```python
from build123d import *

# Parameters (mm, degrees)
F2_DEPTH       = 70
F4_D           = 3.5
F4_CSINK_D     = 7
F4_CSINK_ANGLE = 90


with BuildPart() as f2:
    # F1 (on Front) → F2 (new body)
    with BuildSketch(Plane.XZ):
        with BuildLine():
            Line((0, 3.2153789857), (0, 0))
            Line((0, 0), (41.3793856046, 0))
            Line((41.3793856046, 0), (41.3793856046, 12.0218454194))
            Line((41.3793856046, 12.0218454194), (37.0459675166, 12.0218454194))
            ThreePointArc((37.0459675166, 12.0218454194), (27.4254767926, 4.7506103835), (17.8049860686, 12.0218454194))
            Line((17.8049860686, 12.0218454194), (13.4715679806, 12.0218454194))
            Line((13.4715679806, 12.0218454194), (13.4715679806, 3.2153789857))
            Line((13.4715679806, 3.2153789857), (0, 3.2153789857))
        make_face()
    extrude(amount=F2_DEPTH)

    # F4 (through all)
    with Locations(Plane.XY.offset(3.2153789857)):
        with Locations((6.7357839903, -20), (6.7357839903, -50)):
            CounterSinkHole(F4_D / 2, F4_CSINK_D / 2, counter_sink_angle=F4_CSINK_ANGLE)


solid = f2.part
```
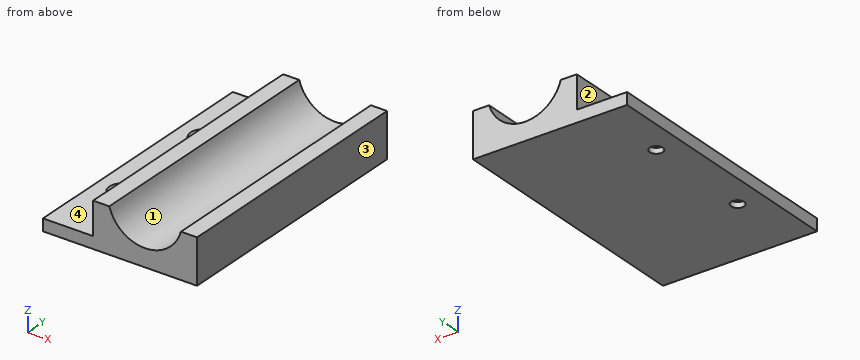
Can you work these out from the model? Positions are in its coordinate system, mm. Face numbers are marked on the shaded views. Round coordinates to 2 decimals unless told otherwise and drop trailing zeros. Loops run counter-clockwise (first coordinate to the right, second up) from the corner with the lowest first, then second, coordinate; pieces in that order, holes last. Notation, with made-up numbers: M -29,78.5 L 28,78.5 A27 cw 28,97.5 Z; hole C 50.5,77.25 d3. An arc over 180 degrees is marked long. Answer in a Markdown table with one row per item.
1. If we section it at C-C, the plane z = 10: Please give me the cut outline in (x, y) (3 decimals).
Established:
| item | result |
|---|---|
| outline | M 13.472,-70 L 18.626,-70 L 18.626,0 L 13.472,0 Z; M 36.225,-70 L 41.379,-70 L 41.379,0 L 36.225,0 Z |
2. If we section it at D-D, the plane x = 24: Please give me the cut outline in (y, z), plus the area to 3 significant figures.
Established:
| item | result |
|---|---|
| outline | M -70,0 L 0,0 L 0,5.36 L -70,5.36 Z |
| area | 375 mm² |
3. If we section it at A-A, the plane y = -20: Please give me the cut outline in (x, z), plus the area to 3 significant figures.
Established:
| item | result |
|---|---|
| outline | M 0,0 L 4.99,0 L 4.99,1.47 L 3.24,3.22 L 0,3.22 Z; M 8.49,0 L 41.38,0 L 41.38,12.02 L 37.05,12.02 A10 cw 17.8,12.02 L 13.47,12.02 L 13.47,3.22 L 10.24,3.22 L 8.49,1.47 Z |
| area | 261 mm² |
4. I'm going to push flat-ended pins straight in: pin 1 Ø4 at (x, y) = (29.5, -51) entering from +Z; pin 2 Ø4.5 at (x, y) = (6.74, -20) entering from +Z; pin 3 Ø4.5 at (y, z) = (-20, 9.5) entering from -X. Where does each tip first touch, or does it pass through?
Established:
| item | result |
|---|---|
| pin 1 | z = 5.62 |
| pin 2 | z = 1.97 |
| pin 3 | x = 13.47 |
5. Please list where these lines run through material, in increasing order: line 1 (X direction, y = -20, z = 0.9); line 2 (Z direction, x = 11, y = -19.5); line 3 (X direction, y = -4.5, z = 3.5). Write a range as from..to.
Established:
| item | result |
|---|---|
| line 1 | 0..4.99, 8.49..41.38 |
| line 2 | 0..3.22 |
| line 3 | 13.47..41.38 |
6. Thinking about a two-plate mould opening in X: for the marked faces 1, 2, 3 and 4, which applies, pulls with the +X half, pulls with the -X half, needs draft (parallel to the pull), parting line crosses it, or undercut?
Established:
| item | result |
|---|---|
| face 1 | undercut |
| face 2 | pulls with the -X half |
| face 3 | pulls with the +X half |
| face 4 | needs draft |
7. If we section it at B-B, the plane z = 5.75: Please give me the cut outline in (x, y), plus the area to 3 significant figures.
Established:
| item | result |
|---|---|
| outline | M 13.47,-70 L 23.07,-70 L 23.07,0 L 13.47,0 Z; M 31.78,-70 L 41.38,-70 L 41.38,0 L 31.78,0 Z |
| area | 1,340 mm² |
